Read the model definition and answer for the solid it produces. Units are mm, in the model's axes. Face numbers are marked on the shaded views. A direction names the side the tool comes from. Coordinates: 2 decimals unless noted, no trailing zeros. Write each loop counter-clockwise with the first axis right and the second up, starting at its lowest first coordinate (ties: lowest second). Pieces come first, ordered by that corner, then holes. Notation, with made-up numbers: (9, 29) -> (29, 29) arc R20 ccw to (29, 51) -> close; hole circle Ø7 at (-30.75, -4.5). An arc over 180 degrees is marked (long way). One line per item, written item: value. Start each with the question number.
1. Find section B-B, the plane z = 20.5. Write down the section's boundary in (x, y), and give its area (3 significant figures).
2. Find section D-D, the plane z = 14. Write down the section's boundary in (x, y).
3. Given P1, Ø5, axis at x = 38.18, z = 38.18, coming from the -Y side; P2, Ø12, axis at x = -18, z = 33, coming from the +Y side; P3, Ø4.5, axis at x = 61, y = 7, coming from the +Z side; P4, Ø6, axis at x = -31.5, y = 3, coming from the -Z side, each flat-ended and moving along its own axis, determine where each tip first touches the part or whether it passes through.
4. Find section C-C, the plane x = 54.5. Write down the section's boundary in (y, z).
5. Consider line 1 along Y through (x, z) = (-40.5, 17); line 2 along X through (y, z) = (15.25, 23); line 3 along X through (y, z) = (18.5, 40). Determine where each line is inside the solid, lowest interval first.
6. For a pull along Y with two mould halves and no side action, classify the marked faces 1, 2, 3 and 4 as pulls with the +Y half, pulls with the -Y half, needs draft (parallel to the pull), parting line crosses it, or undercut.
7. Find section A-A, the plane y = 10. Write down the section's boundary in (x, z), and give its area (3 significant figures).
8. For the marked faces 5 and 6, determine the directions among +Z, -Z, +X, -X, +Y, -Y from which every point of the face is accessible in a straight line to the end or side of a thin tool.
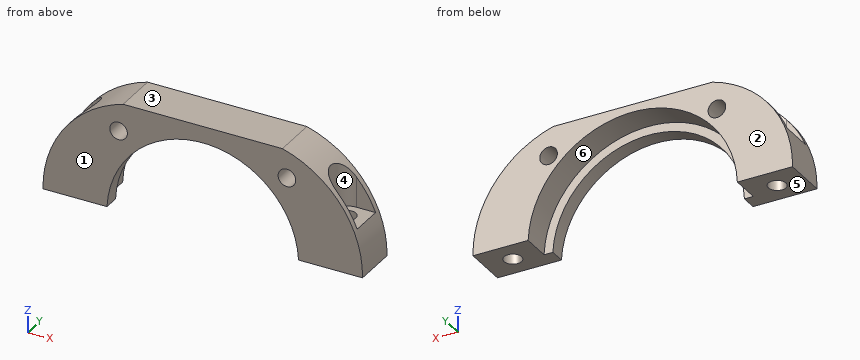
```python
from build123d import *

# Parameters (mm, degrees)
SKETCH1_R           = 62.5
SKETCH1_R_2         = 43.5
BOSS_EXTRUDE1_DEPTH = 20
SKETCH2_R           = 47.5
CUT_EXTRUDE1_DEPTH  = 13
SKETCH3_R           = 4
CUT_EXTRUDE2_DEPTH  = 91.622844802
SKETCH4_W           = 150
SKETCH4_H           = 64.5
SKETCH4_W_2         = 72.256487598
SKETCH4_H_2         = 11.5
CUT_EXTRUDE3_DEPTH  = 91.622844802
BOSS_EXTRUDE4_DEPTH = 20
SKETCH7_R           = 4
CUT_EXTRUDE4_DEPTH  = 90.742875716
SKETCH8_R           = 4
CUT_EXTRUDE5_DEPTH  = 90.742875874
CUT_EXTRUDE6_START  = -20
SKETCH12_W          = 2.494942127
SKETCH12_H          = 15
SKETCH12_R          = 7.5
SKETCH12_R_2        = 4
CUT_EXTRUDE6_DEPTH  = 70.742875874


with BuildPart() as part:
    # Sketch1 → Boss-Extrude1 (new body)
    with BuildSketch(Plane(origin=(0, 0, 0), x_dir=(1, 0, 0), z_dir=(0, 1, 0))):
        with Locations(Location((0, 0, 0), (0, 0, 270))):
            Circle(SKETCH1_R)
        with Locations(Location((0, 0, 0), (0, 0, 270))):
            Circle(SKETCH1_R_2, mode=Mode.SUBTRACT)
    extrude(amount=BOSS_EXTRUDE1_DEPTH)

    # Sketch2 → Cut-Extrude1 (cut)
    with BuildSketch(Plane(origin=(0, 20, 0), x_dir=(1, 0, 0), z_dir=(0, 1, 0))):
        with Locations(Location((0, 0, 0), (0, 0, 270))):
            Circle(SKETCH2_R)
    extrude(amount=-CUT_EXTRUDE1_DEPTH, mode=Mode.SUBTRACT)

    # Sketch3 → Cut-Extrude2 (cut, through all)
    with BuildSketch(Plane(origin=(0, 20, 0), x_dir=(1, 0, 0), z_dir=(0, 1, 0))):
        with Locations(Location((38.183766184, 38.183766184, 0), (0, 0, 270))):
            Circle(SKETCH3_R)
        with Locations(Location((38.183766184, -38.183766184, 0), (0, 0, 270))):
            Circle(SKETCH3_R)
        with Locations(Location((-38.183766184, -38.183766184, 0), (0, 0, 270))):
            Circle(SKETCH3_R)
        with Locations(Location((-38.183766184, 38.183766184, 0), (0, 0, 270))):
            Circle(SKETCH3_R)
    extrude(amount=-CUT_EXTRUDE2_DEPTH, mode=Mode.SUBTRACT)

    # Sketch4 → Cut-Extrude3 (cut, through all)
    with BuildSketch(Plane(origin=(0, 20, 0), x_dir=(1, 0, 0), z_dir=(0, 1, 0))):
        with Locations((0, 30.25)):
            Rectangle(SKETCH4_W, SKETCH4_H)
        with Locations((0, -56.75)):
            Rectangle(SKETCH4_W_2, SKETCH4_H_2)
    extrude(amount=-CUT_EXTRUDE3_DEPTH, mode=Mode.SUBTRACT)

    # Sketch6 → Boss-Extrude4 (add, through all)
    with BuildSketch(Plane(origin=(0, 20, 0), x_dir=(1, 0, 0), z_dir=(0, 1, 0))):
        with BuildLine():
            Line((-62.467991804, -2), (-72.467991804, -2))
            ThreePointArc((-72.467991804, -2), (-62.636910051, -32.684277735), (-36.128243799, -51))
            ThreePointArc((-36.128243799, -51), (-55.050471558, -29.592154049), (-62.467991804, -2))
        make_face()
        with BuildLine():
            ThreePointArc((62.467991804, -2), (55.050471558, -29.592154049), (36.128243799, -51))
            ThreePointArc((36.128243799, -51), (62.636910051, -32.684277735), (72.467991804, -2))
            Line((72.467991804, -2), (62.467991804, -2))
        make_face()
    extrude(amount=-BOSS_EXTRUDE4_DEPTH)

    # Sketch7 → Cut-Extrude4 (cut, through all)
    with BuildSketch(Plane(origin=(0, 0, 2), x_dir=(-1, 0, 0), z_dir=(0, 0, -1))):
        with Locations((-59.962933931, 10)):
            Circle(SKETCH7_R)
    extrude(amount=-CUT_EXTRUDE4_DEPTH, mode=Mode.SUBTRACT)

    # Sketch8 → Cut-Extrude5 (cut, through all)
    with BuildSketch(Plane(origin=(0, 0, 2), x_dir=(-1, 0, 0), z_dir=(0, 0, -1))):
        with Locations((59.962933931, 10)):
            Circle(SKETCH8_R)
    extrude(amount=-CUT_EXTRUDE5_DEPTH, mode=Mode.SUBTRACT)

    # Sketch12 → Cut-Extrude6 (cut, through all)
    # profile 1 of 3: a face of its own
    with BuildSketch(Plane(origin=(0, 0, 2), x_dir=(-1, 0, 0), z_dir=(0, 0, -1)).offset(CUT_EXTRUDE6_START)):
        with Locations((73.715462868, 10)):
            Rectangle(SKETCH12_W, SKETCH12_H)
    # profile 2 of 3: a face of its own
    with BuildSketch(Plane(origin=(0, 0, 2), x_dir=(-1, 0, 0), z_dir=(0, 0, -1)).offset(CUT_EXTRUDE6_START)):
        with Locations((59.962933931, 10)):
            Circle(SKETCH12_R)
        with Locations((59.962933931, 10)):
            Circle(SKETCH12_R_2, mode=Mode.SUBTRACT)
    # profile 3 of 3: a face of its own
    with BuildSketch(Plane(origin=(0, 0, 2), x_dir=(-1, 0, 0), z_dir=(0, 0, -1)).offset(CUT_EXTRUDE6_START)):
        with BuildLine():
            Line((59.962933931, 2.5), (72.467991804, 2.5))
            Line((72.467991804, 2.5), (72.467991804, 17.5))
            Line((72.467991804, 17.5), (59.962933931, 17.5))
            ThreePointArc((59.962933931, 17.5), (65.26623479, 15.303300859), (67.462933931, 10))
            ThreePointArc((67.462933931, 10), (65.26623479, 4.696699141), (59.962933931, 2.5))
        make_face()
    cut_extrude6 = extrude(amount=-CUT_EXTRUDE6_DEPTH, mode=Mode.SUBTRACT)

    # Mirror1: Cut-Extrude6 across plane
    add(cut_extrude6.mirror(Plane(origin=(0, 0, 0), x_dir=(0, 0, 1), z_dir=(1, 0, 0))), mode=Mode.SUBTRACT)


solid = part.part
```
Answer block:
1. outline: (-69.28, 0) -> (-38.37, 0) -> (-38.37, 7) -> (-42.85, 7) -> (-42.85, 20) -> (-69.28, 20) -> close; (38.37, 0) -> (69.28, 0) -> (69.28, 20) -> (42.85, 20) -> (42.85, 7) -> (38.37, 7) -> close; hole circle Ø8 at (-59.96, 10); hole circle Ø8 at (59.96, 10)
1. area: 1,020 mm2
2. outline: (-71.23, 0) -> (-41.19, 0) -> (-41.19, 7) -> (-45.39, 7) -> (-45.39, 20) -> (-71.23, 20) -> close; (41.19, 0) -> (71.23, 0) -> (71.23, 20) -> (45.39, 20) -> (45.39, 7) -> (41.19, 7) -> close; hole circle Ø8 at (-59.96, 10); hole circle Ø8 at (59.96, 10)
3. P1: passes through
3. P2: stops at y = 7
3. P3: stops at z = 22
3. P4: stops at z = 26.5
4. outline: (0, 2) -> (20, 2) -> (20, 41.3) -> (15.14, 41.3) -> (15.14, 22) -> (4.86, 22) -> (4.86, 41.3) -> (0, 41.3) -> close
5. line 1: y = 0 to 7
5. line 2: x = -54.61 to -41.56, 41.56 to 54.61
5. line 3: x = -56 to -41.75, -34.62 to -25.62, 25.62 to 34.62, 41.75 to 56
6. face 1: pulls with the -Y half
6. face 2: pulls with the +Y half
6. face 3: needs draft
6. face 4: undercut
7. outline: (-72.47, 2) -> (-63.96, 2) -> (-63.96, 22) -> (-68.68, 22) arc R50 ccw to start; (-55.96, 2) -> (-47.46, 2) arc R47.5 cw to (47.46, 2) -> (55.96, 2) -> (55.96, 22) -> (52.46, 22) -> (52.46, 42.91) arc R50 ccw to (36.13, 51) -> (-36.13, 51) arc R50 ccw to (-52.46, 42.91) -> (-52.46, 22) -> (-55.96, 22) -> close; (63.96, 2) -> (72.47, 2) arc R50 ccw to (68.68, 22) -> (63.96, 22) -> close; hole circle Ø8 at (-38.18, 38.18); hole circle Ø8 at (38.18, 38.18)
7. area: 2,010 mm2
8. face 5: -Z, +X, -X, +Y, -Y
8. face 6: -Z, +Y
